```python
from build123d import *

# Parameters (mm, degrees)
BOSS_EXTRUDE1_DEPTH     = 50
CUT_EXTRUDE1_DEPTH      = 1.35
CUT_EXTRUDE1_DEPTH_BACK = 1.35
SKETCH3_W               = 40
SKETCH3_H               = 20
CUT_EXTRUDE2_DEPTH      = 52.612698372
FILLET1_R               = 0.5
FILLET2_R               = 2


with BuildPart() as part:
    # Sketch1 → Boss-Extrude1 (new body)
    with BuildSketch(Plane.XY):
        Polygon((-23.914213562, -1), (-1.560660172, -1), (-1.560660172, 21.353553391), (-4.389087297, 18.525126266), (-7.217514421, 21.353553391), (1.974873734, 30.545941546), (4.803300859, 27.717514421), (0.439339828, 23.353553391), (0.439339828, -3), (-25.914213562, -3), (-30.278174593, -7.363961031), (-33.106601718, -4.535533906), (-23.914213562, 4.656854249), (-21.085786438, 1.828427125), align=None)
    extrude(amount=-BOSS_EXTRUDE1_DEPTH)

    # Sketch2 → Cut-Extrude1 (cut, two sides)
    with BuildSketch(Plane(origin=(-12.871320344, 12.871320344, 0), x_dir=(0.707106781, 0.707106781, 0), z_dir=(-0.707106781, 0.707106781, 0))) as cut_extrude1_sk:
        with BuildLine():
            Line((19.925, 1.925), (22.995689014, 1.925))
            Line((22.995689014, 1.925), (22.995689014, 8.225))
            Line((22.995689014, 8.225), (19.925, 8.225))
            ThreePointArc((19.925, 8.225), (16.775, 5.075), (19.925, 1.925))
        make_face()
        with BuildLine():
            Line((19.925, 41.775), (22.995689014, 41.775))
            Line((22.995689014, 41.775), (22.995689014, 48.075))
            Line((22.995689014, 48.075), (19.925, 48.075))
            ThreePointArc((19.925, 48.075), (16.775, 44.925), (19.925, 41.775))
        make_face()
        with BuildLine():
            Line((-19.925, 1.925), (-26.617009358, 1.925))
            Line((-26.617009358, 1.925), (-26.617009358, 8.225))
            Line((-26.617009358, 8.225), (-19.925, 8.225))
            ThreePointArc((-19.925, 8.225), (-16.775, 5.075), (-19.925, 1.925))
        make_face()
        with BuildLine():
            Line((-19.925, 41.775), (-26.617009358, 41.775))
            Line((-26.617009358, 41.775), (-26.617009358, 48.075))
            Line((-26.617009358, 48.075), (-19.925, 48.075))
            ThreePointArc((-19.925, 48.075), (-16.775, 44.925), (-19.925, 41.775))
        make_face()
    extrude(amount=CUT_EXTRUDE1_DEPTH, mode=Mode.SUBTRACT)
    extrude(cut_extrude1_sk.sketch, amount=-CUT_EXTRUDE1_DEPTH_BACK, mode=Mode.SUBTRACT)

    # Sketch3 → Cut-Extrude2 (cut, through all)
    with BuildSketch(Plane(origin=(16.26040764, 16.26040764, 0), x_dir=(0, 0, -1), z_dir=(0.707106781, 0.707106781, 0))):
        with Locations((25, 3.202795796)):
            Rectangle(SKETCH3_W, SKETCH3_H)
    extrude(amount=-CUT_EXTRUDE2_DEPTH, mode=Mode.SUBTRACT)

    # Fillet1
    fillet1_edges = [part.edges().sort_by_distance(p)[0] for p in [
        (-1.560660172, 21.353553391, -25),
        (-23.914213562, -1, -25),
    ]]
    fillet(fillet1_edges, radius=FILLET1_R)

    # Fillet2
    fillet2_edges = [part.edges().sort_by_distance(p)[0] for p in [
        (0.439339828, -3, -47.5),
        (0.439339828, -3, -2.5),
    ]]
    fillet(fillet2_edges, radius=FILLET2_R)


solid = part.part
```
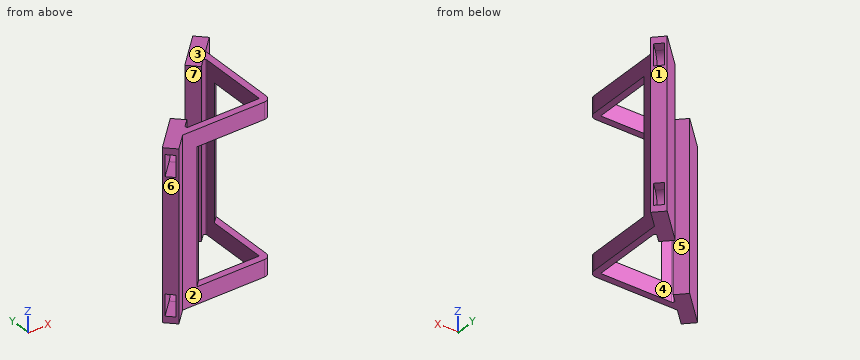
Check sheet for the modelled part. Datum: model origin and axes. Units: mm. Face numbers are marked on the shaded views. A direction names the side the tool comes from. Coordinates: 2 decimals unless noted, no trailing zeros. Order: outer loops, then holes, each group sorted by start corner. A loop starts at its lowest first (then second) coordinate and runs counter-clockwise, first axis right, second up. Notation, with made-up numbers: (36, 81.5) -> (42, 81.5) arc R25 ccw to (42, 110.5) -> close; hole circle Ø5 at (20, -1). An arc over 180 degrees is marked (long way). Write each question's results on one line, items separated by ' | '. Start each with the question number.
1) Depth check by flat-ended pin: pin 1 (17 mm diameter, centred on y = 15, z = -17, fed in from -X); pin 2 (10 mm diameter, centred on y = 6.5, z = -24, fed in from -X); pin 3 (12 mm diameter, centred on x = -11.5, z = -23, fed in from -Y). Enter the tip coordinate at first touch or a pass-through.
2) Section check B-B (z = -34.5). Enter the section's corners in (x, y).
3) Material ranges on line 1 along Z through (x, y) = (-0.5, 3); line 2 along X through (y, z) = (20, -38); line 3 along X through (y, z) = (25, -45), recorded low to high.
4) Set-up check for the marked faces 5, 6 and 7: record each of +Z, -Z, +X, -X, +Y, -Y from which the full face is reachable in a straight line by a thin tool's end or side.
5) Draft check along Y on the marked faces 1, 2, 3 and 4. Enter one of: pulls with the +Y half, pulls with the -Y half, needs draft (parallel to the pull), parting line crosses it, or undercut.
6) Section check D-D (x = -29). Enter the section's corners in (y, z) (3 decimals), and give its area (3 significant figures).
7) Section check C-C (y = 11). Enter the section's corners in (x, z), and give its area (3 significant figures).
8) Section check A-A (x = -13.5). Enter the section's corners in (y, z).
Checked values:
1) pin 1: x = -7.22 | pin 2: x = -27.07 | pin 3: y = 19.64
2) outline: (-33.11, -4.54) -> (-30.28, -7.36) -> (-25.91, -3) -> (-21.67, -3) -> (-19.67, -1) -> (-22.71, -1) arc R0.5 cw to (-23.06, -0.15) -> (-21.09, 1.83) -> (-23.91, 4.66) -> close; (-7.22, 21.35) -> (-4.39, 18.53) -> (-2.41, 20.5) arc R0.5 cw to (-1.56, 20.15) -> (-1.56, 17.11) -> (0.44, 19.11) -> (0.44, 23.35) -> (4.8, 27.72) -> (1.97, 30.55) -> close
3) line 1: -50 to -45, -5 to 0 | line 2: -5.86 to -2.91, -1.56 to 0.44 | line 3: -3.57 to -1.28, 1.17 to 2.09
4) face 5: +Z, -Z, +Y | face 6: +Z, -Z, -X, -Y | face 7: +Z, -Z, -X
5) face 1: pulls with the +Y half | face 2: pulls with the -Y half | face 3: needs draft | face 4: undercut
6) outline: (-6.086, -50) -> (-0.429, -50) -> (-0.429, 0) -> (-6.086, 0) -> close; hole (-5.167, -48.075) -> (-1.348, -48.075) -> (-1.348, -41.775) -> (-5.167, -41.775) -> close; hole (-5.167, -8.225) -> (-1.348, -8.225) -> (-1.348, -1.925) -> (-5.167, -1.925) -> close | area: 235 mm²
7) outline: (-1.56, -50) -> (0.44, -50) -> (0.44, -45) -> (-1.56, -45) -> close; (-1.56, -5) -> (0.44, -5) -> (0.44, 0) -> (-1.56, 0) -> close | area: 20.0 mm²
8) outline: (-3, -50) -> (-1, -50) -> (-1, -45) -> (-3, -45) -> close; (-3, -5) -> (-1, -5) -> (-1, 0) -> (-3, 0) -> close
